from build123d import *

# Parameters (mm, degrees)
SKETCH1_R                = 125
BOSS_EXTRUDE1_DEPTH      = 20
SKETCH2_W                = 106
SKETCH2_H                = 135
BOSS_EXTRUDE2_DEPTH      = 160
SKETCH5_R                = 20
CUT_EXTRUDE2_DEPTH       = 283.327823638
SKETCH6_W                = 76
SKETCH6_H                = 135
CUT_EXTRUDE3_DEPTH       = 130
SKETCH7_W                = 106
SKETCH7_H                = 135
SKETCH7_R                = 25
CUT_EXTRUDE5_DEPTH       = 29
SKETCH10_W               = 106
SKETCH10_H               = 135
SKETCH10_R               = 47.5
BOSS_EXTRUDE4_DEPTH      = 5
SKETCH11_R               = 2.5
CUT_EXTRUDE6_DEPTH       = 253.289516231
SKETCH12_R               = 2.5
CUT_EXTRUDE7_DEPTH       = 253.289516231
SKETCH13_R               = 5
CUT_EXTRUDE8_DEPTH       = 5
CUT_EXTRUDE10_REACH      = 237.767
SKETCH14_R               = 94.455144731
SKETCH14_R_2             = 75
SKETCH15_W               = 15
SKETCH15_H               = 106.131993292
CUT_EXTRUDE11_DEPTH      = 20
CUT_EXTRUDE12_DEPTH      = 274.119021674
CUT_EXTRUDE12_DEPTH_BACK = 274.119021674
CUT_EXTRUDE13_DEPTH      = 4


with BuildPart() as part:
    # Sketch1 → Boss-Extrude1 (new body)
    with BuildSketch(Plane(origin=(0, 0, 0), x_dir=(1, 0, 0), z_dir=(0, 1, 0))):
        with Locations(Location((0, 0, 0), (0, 0, 270))):
            Circle(SKETCH1_R)
    extrude(amount=BOSS_EXTRUDE1_DEPTH)

    # Sketch2 → Boss-Extrude2 (add)
    with BuildSketch(Plane(origin=(0, 20, 0), x_dir=(1, 0, 0), z_dir=(0, 1, 0))):
        Rectangle(SKETCH2_W, SKETCH2_H)
    extrude(amount=BOSS_EXTRUDE2_DEPTH)

    # Sketch5 → Cut-Extrude2 (cut, through all)
    with BuildSketch(Plane(origin=(53, 0, 0), x_dir=(0, 0, -1), z_dir=(1, 0, 0))):
        with Locations((0, 110)):
            Circle(SKETCH5_R)
    extrude(amount=-CUT_EXTRUDE2_DEPTH, mode=Mode.SUBTRACT)

    # Sketch6 → Cut-Extrude3 (cut)
    with BuildSketch(Plane.XZ):
        Rectangle(SKETCH6_W, SKETCH6_H)
    extrude(amount=-CUT_EXTRUDE3_DEPTH, mode=Mode.SUBTRACT)

    # Sketch7 → Cut-Extrude5 (cut)
    with BuildSketch(Plane(origin=(0, 180, 0), x_dir=(1, 0, 0), z_dir=(0, 1, 0))):
        Rectangle(SKETCH7_W, SKETCH7_H)
        with Locations(Location((0, 0, 0), (0, 0, 270))):
            Circle(SKETCH7_R, mode=Mode.SUBTRACT)
    extrude(amount=-CUT_EXTRUDE5_DEPTH, mode=Mode.SUBTRACT)

    # Sketch10 → Boss-Extrude4 (add)
    with BuildSketch(Plane(origin=(0, 151, 0), x_dir=(1, 0, 0), z_dir=(0, 1, 0))):
        Rectangle(SKETCH10_W, SKETCH10_H)
        with Locations(Location((0, 0, 0), (0, 0, 270))):
            Circle(SKETCH10_R, mode=Mode.SUBTRACT)
    extrude(amount=BOSS_EXTRUDE4_DEPTH)

    # Sketch11 → Cut-Extrude6 (cut, through all)
    with BuildSketch(Plane(origin=(0, 0, 0), x_dir=(-1, 0, 0), z_dir=(0, -1, 0))):
        with Locations(Location((83.502937015, 0, 0), (0, 0, 90))):
            Circle(SKETCH11_R)
        with Locations(Location((-83.502937015, 0, 0), (0, 0, 90))):
            Circle(SKETCH11_R)
        with Locations(Location((83.502937015, -30, 0), (0, 0, 90))):
            Circle(SKETCH11_R)
        with Locations(Location((83.502937015, 30, 0), (0, 0, 90))):
            Circle(SKETCH11_R)
        with Locations(Location((-83.502937015, 30, 0), (0, 0, 90))):
            Circle(SKETCH11_R)
        with Locations(Location((-83.502937015, -30, 0), (0, 0, 90))):
            Circle(SKETCH11_R)
    extrude(amount=-CUT_EXTRUDE6_DEPTH, mode=Mode.SUBTRACT)

    # Sketch12 → Cut-Extrude7 (cut, through all)
    with BuildSketch(Plane(origin=(0, 0, 0), x_dir=(-1, 0, 0), z_dir=(0, -1, 0))):
        with Locations(Location((0, 87.5, 0), (0, 0, 90))):
            Circle(SKETCH12_R)
        with Locations(Location((75.777222831, 43.75, 0), (0, 0, 90))):
            Circle(SKETCH12_R)
        with Locations(Location((75.777222831, -43.75, 0), (0, 0, 90))):
            Circle(SKETCH12_R)
        with Locations(Location((0, -87.5, 0), (0, 0, 90))):
            Circle(SKETCH12_R)
        with Locations(Location((-75.777222831, -43.75, 0), (0, 0, 90))):
            Circle(SKETCH12_R)
        with Locations(Location((-75.777222831, 43.75, 0), (0, 0, 90))):
            Circle(SKETCH12_R)
    extrude(amount=-CUT_EXTRUDE7_DEPTH, mode=Mode.SUBTRACT)

    # Sketch13 → Cut-Extrude8 (cut)
    with BuildSketch(Plane(origin=(0, 0, 0), x_dir=(-1, 0, 0), z_dir=(0, -1, 0))):
        with Locations(Location((0, -87.5, 0), (0, 0, 90))):
            Circle(SKETCH13_R)
        with Locations(Location((-75.777222831, -43.75, 0), (0, 0, 90))):
            Circle(SKETCH13_R)
        with Locations(Location((-75.777222831, 43.75, 0), (0, 0, 90))):
            Circle(SKETCH13_R)
        with Locations(Location((0, 87.5, 0), (0, 0, 90))):
            Circle(SKETCH13_R)
        with Locations(Location((75.777222831, 43.75, 0), (0, 0, 90))):
            Circle(SKETCH13_R)
        with Locations(Location((75.777222831, -43.75, 0), (0, 0, 90))):
            Circle(SKETCH13_R)
    extrude(amount=-CUT_EXTRUDE8_DEPTH, mode=Mode.SUBTRACT)

    # Cut-Extrude10: up to this face of the body (flat: up to its plane)
    cut_extrude10_end = Plane(part.part.faces().sort_by_distance((0, 20, -121.464466094))[0])
    # Sketch14 → Cut-Extrude10 (cut, up to the picked face)
    with BuildSketch(Plane(origin=(0, 156, 0), x_dir=(1, 0, 0), z_dir=(0, 1, 0)), mode=Mode.PRIVATE) as cut_extrude10_sk1:
        Circle(SKETCH14_R)
        Circle(SKETCH14_R_2, mode=Mode.SUBTRACT)
    cut_extrude10_tool1 = split(extrude(cut_extrude10_sk1.sketch, amount=-CUT_EXTRUDE10_REACH, mode=Mode.PRIVATE), bisect_by=cut_extrude10_end, keep=Keep.BOTH, mode=Mode.PRIVATE)
    add(cut_extrude10_tool1.solids().sort_by(Axis((-91.78355, 156, 0), (0, -1, 0)))[0], mode=Mode.SUBTRACT)

    # Sketch15 → Cut-Extrude11 (cut)
    with BuildSketch(Plane(origin=(0, 20, 0), x_dir=(1, 0, 0), z_dir=(0, 1, 0))):
        with Locations((-60.5, 0)):
            Rectangle(SKETCH15_W, SKETCH15_H)
    extrude(amount=-CUT_EXTRUDE11_DEPTH, mode=Mode.SUBTRACT)

    # Sketch16 → Cut-Extrude12 (cut, two sides: drawn at the far end of the back side and taken through both)
    with BuildSketch(Plane(origin=(-38, 0, 0), x_dir=(0, 0, -1), z_dir=(1, 0, 0)).offset(-CUT_EXTRUDE12_DEPTH_BACK)):
        with BuildLine():
            Line((-15, 72.5), (15, 72.5))
            ThreePointArc((15, 72.5), (17.5, 70), (15, 67.5))
            Line((15, 67.5), (-15, 67.5))
            ThreePointArc((-15, 67.5), (-17.5, 70), (-15, 72.5))
        make_face()
    extrude(amount=CUT_EXTRUDE12_DEPTH + CUT_EXTRUDE12_DEPTH_BACK, mode=Mode.SUBTRACT)

    # Sketch17 → Cut-Extrude13 (cut)
    with BuildSketch(Plane.ZY.offset(53)):
        with BuildLine():
            Line((-15, 74), (15, 74))
            ThreePointArc((15, 74), (19, 70), (15, 66))
            Line((15, 66), (-15, 66))
            ThreePointArc((-15, 66), (-19, 70), (-15, 74))
        make_face()
    cut_extrude13 = extrude(amount=-CUT_EXTRUDE13_DEPTH, mode=Mode.SUBTRACT)

    # Mirror1: Cut-Extrude13 across plane
    add(cut_extrude13.mirror(Plane(origin=(0, 0, 0), x_dir=(0, 0, 1), z_dir=(1, 0, 0))), mode=Mode.SUBTRACT)


solid = part.part
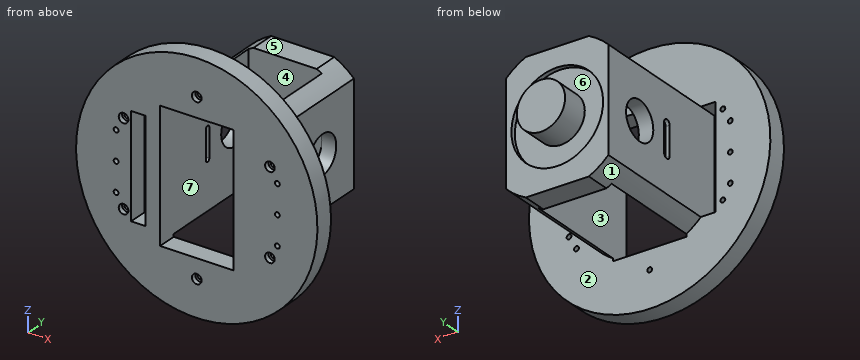
Check sheet for the modelled part. Datum: model origin and axes. Units: mm. Face numbers are marked on the shaded views. A direction names the side the tool comes from. Give positions to 0.01 mm unless a question says otherwise; leave off trailing zeros. Order: outer loops, then holes, each group sorted by start corner. A loop starts at its lowest first (then second) coordinate and runs counter-clockwise, first axis right, second up. Notation, with made-up numbers: M -17,28.5 L 15,28.5 A4 cw 15,32.5 Z; hole C 35.25,59 d6. An arc over 180 degrees is marked long. Answer as CSV lines item,"result". Start each with the question number.
Item 1: Gauge pin test, flat ends, axial feed: P1, Ø4, axis at x = 27.5, z = 84, coming from the -Y side; P2, Ø1.5, axis at y = 85.5, z = 36, coming from the -X side; P3, Ø8, axis at x = 83.5, z = -30, coming from the +Y side; P4, Ø12, axis at x = 31, z = -23.5, coming from the +Y side. Record the tip position at first contact, or that the pin passes through.
Item 2: Thickness scan on line 1 (X direction, y = 9, z = 0); line 2 (X direction, y = 152, z = 0); line 3 (X direction, y = 68.5, z = 31). Record the ranges inside material, lowest first. Write a range as [from, to].
Item 3: Cross-section at C-C on z = 7. State how many separate pieces and enclosed holes the cut face has, plus the area to 3 significant figures.
Item 4: Cross-section at A-A on y = 110. Enter the section's corners in (x, z).
Item 5: Mould release check, pull along X, two halves, no side actions. Record for the marked faces 1, 2 and 3: +X half, -X half, draft (parallel to the pull), parting line (faces both ways), or undercut.
Item 6: Tool access check on the marked faces 4, 5, 6 and 7. Record the directions out of +Z, -Z, +X, -X, +Y, -Y that give a thin tool (end or side, any length) a straight path to the whole face; none if there is none.
Item 7: Cross-section at B-B on y = 62. Enter the section's corners in (x, z).
Item 8: Cross-section at D-D on x = 96.5. Enter the section's corners in (y, z), plus the area to 3 significant figures.
Established:
1,P1,"stops at y = 0"
1,P2,"stops at x = -53"
1,P3,"stops at y = 20"
1,P4,"stops at y = 151"
2,line 1,"x = [-125, -86], [-81, -68], [-53, -38], [38, 81], [86, 125]"
2,line 2,"x = [-53, -47.5], [-25, 25], [47.5, 53]"
2,line 3,"x = [-53, -38], [38, 53]"
3,separate pieces,"6"
3,enclosed holes,"0"
3,area,"8,850 mm^2"
4,outline,"M -53,-53.07 A75 ccw -38,-64.66 L -38,-20 L -53,-20 Z; M -53,20 L -38,20 L -38,64.66 A75 ccw -53,53.07 Z; M 38,-64.66 A75 ccw 53,-53.07 L 53,-20 L 38,-20 Z; M 38,20 L 53,20 L 53,53.07 A75 ccw 38,64.66 Z"
5,face 1,"-X half"
5,face 2,"draft"
5,face 3,"undercut"
6,face 4,"+Z, -Z, -Y"
6,face 5,"+Z, +X, -X, +Y"
6,face 6,"+Y"
6,face 7,"-Y"
7,outline,"M -53,-53.07 A75 ccw -38,-64.66 L -38,64.66 A75 ccw -53,53.07 Z; M 38,-64.66 A75 ccw 53,-53.07 L 53,53.07 A75 ccw 38,64.66 Z"
8,outline,"M 0,-79.45 L 20,-79.45 L 20,79.45 L 0,79.45 Z"
8,area,"3,180 mm^2"
